The listing builds one solid part. Answer for the finished solid, in the listing's coordinates (mm). A direction names the side the tool comes from. Coordinates: 2 decimals unless noted, no trailing zeros. Write each loop counter-clockwise with the first axis right and the second up, starting at its lowest first coordinate (ties: lowest second). Pieces come first, ordered by that corner, then holes.
```python
from build123d import *

# Parameters (mm, degrees)
SKETCH1_R           = 22.225
BOSS_EXTRUDE1_DEPTH = 95.25
SKETCH6_R           = 19.05
SKETCH6_R_2         = 6.35
CUT_EXTRUDE1_DEPTH  = 88.9
CUT_EXTRUDE1_DRAFT  = -1


with BuildPart() as part:
    # Sketch1 → Boss-Extrude1 (new body)
    with BuildSketch(Plane(origin=(0, 0, 0), x_dir=(1, 0, 0), z_dir=(0, 1, 0))):
        with Locations(Location((0, 0, 0), (0, 0, 270))):
            Circle(SKETCH1_R)
    extrude(amount=BOSS_EXTRUDE1_DEPTH)


with BuildPart() as cut_extrude1_tool:
    # Sketch6 → Cut-Extrude1 (with draft: the straight prism first)
    with BuildSketch(Plane(origin=(0, 95.25, 0), x_dir=(1, 0, 0), z_dir=(0, 1, 0))):
        Circle(SKETCH6_R)
        Circle(SKETCH6_R_2, mode=Mode.SUBTRACT)
    extrude(amount=-CUT_EXTRUDE1_DEPTH)
    # Cut-Extrude1: the draft: its side faces are tilted about the plane it starts from
    cut_extrude1_sides = [cut_extrude1_tool.faces().sort_by_distance(p)[0] for p in [
        (-19.05, 50.8, 0),
        (-6.35, 50.8, 0),
    ]]
    draft(cut_extrude1_sides, Plane(origin=(0, 95.25, 0), x_dir=(1, 0, 0), z_dir=(0, 1, 0)), CUT_EXTRUDE1_DRAFT)


with BuildPart() as part_1:
    add(part.part)

    # Cut-Extrude1: cut by cut_extrude1_tool
    add(cut_extrude1_tool.part, mode=Mode.SUBTRACT)


solid = part_1.part
```
(1) Section A-A, the plane y = 56.5 is taken. Write down the section's boundary in (x, z) (3 decimals), plus the area to 3 significant figures.
(2) Which of the six approach directions +Z, -Z, +X, -X, +Y, -Y give full straight-line access (tool end or side, diameter ignored) to faces 1 (the conical face through (-14.51, 51.422, 11.126)), 2 (the flat face through (10, 95.25, 16.4))?
(3) Find the intervals of material crossed by probe 1 along X at (y, z) = (6.5, 4); probe 2 along X at (y, z) = (64, -5); probe 3 along Y at (x, z) = (10, 4), in increasing order.
(4) For a pull along X with two mould halves and no side action, classify faces 3 (the flat face through (0, 95.25, 0)), 4 (the cylindrical face through (18.74, 46.96, 11.95)), 5 (the flat face through (8, 6.35, 4)) as pulls with the +X half, pulls with the -X half, needs draft (parallel to the pull), parting line crosses it, or undercut.
(5) Each of these flat-tipped pins is pushed along its axis until it touches: pin 1 (4 mm diameter, centred on x = -11.5, y = 58.5, fed in from +Z); pin 2 (5 mm diameter, centred on y = 32.5, z = -17.5, fed in from -X); pin 3 (12 mm diameter, centred on y = 57.5, z = 2, fed in from -X) (3 decimals); pin 4 (6 mm diameter, centred on x = -3.5, z = 17, fed in from +Y). Where does it stop, or does it pass through?
Solution:
1. outline: circle Ø44.45 at (0, 0); circle Ø14.053 at (0, 0); hole circle Ø36.747 at (0, 0)
1. area: 646 mm2
2. face 1: +Y
2. face 2: +Z, -Z, +X, -X, +Y
3. probe 1: x = -21.86 to -17.04, -6.81 to 6.81, 17.04 to 21.86
3. probe 2: x = -21.66 to -17.82, -4.75 to 4.75, 17.82 to 21.66
3. probe 3: y = 0 to 6.35
4. face 3: needs draft
4. face 4: parting line crosses it
4. face 5: undercut
5. pin 1: stops at z = 20.09
5. pin 2: stops at x = -16.4
5. pin 3: stops at x = -22.225
5. pin 4: stops at y = 95.25
